Autodesk Inventor part; units mm, degrees
ref_plane "YZ Plane" through (0, 0, 0) normal (1, 0, 0) x (0, 1, 0)
ref_plane "XZ Plane" through (0, 0, 0) normal (0, 1, 0) x (-1, 0, 0)
ref_plane "XY Plane" through (0, 0, 0) normal (0, 0, 1) x (1, 0, 0)
sketch "Sketch1" plane through (0, 0, 0) normal (1, 0, 0) x (0, 1, 0)
  line L0 (6.1324, -19.2794) -> (-5.8676, -19.2794)
  line L1 (-5.8676, -19.2794) -> (-5.8676, -43.2794)
  line L2 (-5.8676, -43.2794) -> (6.1324, -43.2794)
  line L3 (6.1324, -43.2794) -> (6.1324, -19.2794)
  point P0 (0, 0)
  dimension "d0" = 12
  dimension "d1" = 24
extrude "Extrusion1" add sketch "Sketch1" along normal blind 1.8
sketch "Sketch2" plane through (1.8, 0, 0) normal (1, 0, 0) x (0, 0, -1)
  circle A0 centre (38.2794, 0.1324) radius 3.5
  line L0 (43.2794, -5.8676) -> (43.2794, 6.1324)
  line L1 (19.2794, -5.8676) -> (43.2794, -5.8676)
  point P0 (0, 0)
  dimension "d4" = 7
  dimension "d5" = 5
  dimension "d6" = 6
extrude "Extrusion2" cut sketch "Sketch2" against normal blind 0.8
sketch "Sketch3" plane through (1.8, 0, 0) normal (1, 0, 0) x (0, 0, -1)
  line L0 (19.2794, 6.1324) -> (19.2794, -5.8676)
  line L1 (43.2794, -5.8676) -> (43.2794, 6.1324)
  line L2 (19.2794, 6.1324) -> (43.2794, 6.1324)
  line L3 (43.2794, 6.1324) -> (43.2794, -5.8676)
  line L4 (43.2794, -5.8676) -> (19.2794, -5.8676)
  line L5 (19.2794, -5.8676) -> (19.2794, 6.1324)
  circle A0 centre (38.2794, 0.1324) radius 3.5
  circle A1 centre (38.2794, 0.1324) radius 3.5
  point P0 (0, 0)
  point P1 (43.2794, 6.1324)
extrude "Extrusion3" add sketch "Sketch3" along normal blind 2.5
sketch "Sketch4" plane through (4.3, 0, 0) normal (1, 0, 0) x (0, 0, -1)
  circle A0 centre (38.2794, 0.1324) radius 3.5
  line L0 (36.7494, 3.2802) -> (22.2595, 1.8824)
  line L1 (36.7494, -3.0155) -> (22.2595, -1.6176)
  arc A1 (22.2595, 1.8824) -> (22.2595, -1.6176) centre (25.2089, 0.1324) ccw
  line L2 (43.2794, 6.1324) -> (19.2794, 6.1324)
  point P0 (0, 0)
  point P1 (21.7794, 0.1324)
  dimension "d15" = 1.53
  dimension "d16" = 1.53
  dimension "d17" = 16.5
  dimension "d18" = 3.5
  dimension "d19" = 6
extrude "Extrusion4" cut sketch "Sketch4" against normal blind 2.5 contours A0 L1 A1 L0
sketch "Sketch5" plane through (0, 0, 0) normal (-1, 0, 0) x (0, 0, 1)
  circle A0 centre (-38.2794, 0.1324) radius 3.5
  circle A1 centre (-38.2794, 0.1324) radius 1.25
  point P0 (0, 0)
  dimension "d22" = 2.5
extrude "Extrusion5" cut sketch "Sketch5" against normal blind 2.5 contours A1
sketch "Sketch6" plane through (4.3, 0, 0) normal (1, 0, 0) x (0, 0, -1)
  line L0 (43.2794, 6.1324) -> (19.2794, 6.1324)
  line L1 (19.2794, -5.8676) -> (43.2794, -5.8676)
  line L2 (19.2794, 6.1324) -> (22.2794, 6.1324)
  line L3 (22.2794, 6.1324) -> (22.2794, -5.8676)
  line L4 (22.2794, -5.8676) -> (19.2794, -5.8676)
  line L5 (19.2794, -5.8676) -> (19.2794, 6.1324)
  point P0 (0, 0)
  point P1 (22.2794, 6.1324)
  dimension "d25" = 3
extrude "Extrusion6" add sketch "Sketch6" along normal blind 45.5
sketch "Sketch7" plane through (0, -5.8676, -19.2794) normal (0, 0, 1) x (1, 0, 0)
  circle A0 centre (39.861, 6) radius 1.5
  line L0 (49.8, 12) -> (49.8, 0)
  line L1 (0, 12) -> (49.8, 12)
  line L2 (0, 12) -> (0, 0)
  point P0 (0, 5.8676)
  dimension "d28" = 3
  dimension "d30" = 6
  dimension "d38" = 39.861
extrude "Extrusion7" cut sketch "Sketch7" against normal blind 40
sketch "Sketch8" plane through (1.8, 0, 0) normal (1, 0, 0) x (0, 0, -1)
  circle A0 centre (25.7794, 0.1324) radius 1
  circle A1 centre (38.2794, 0.1324) radius 1.25
  point P0 (0, 0)
  dimension "d33" = 2
  dimension "d34" = 12.5
  dimension "d35" = 0
extrude "Extrusion8" cut sketch "Sketch8" against normal blind 10 contours A0
properties part number "18_2"
Part model, mm, in its own coordinate system. A direction names the side the tool comes from. Round coordinates to 2 decimals unless told otherwise and drop trailing zeros. Loops run counter-clockwise (first coordinate to the right, second up) from the corner with the lowest first, then second, coordinate; pieces in that order, holes last. Notation, with made-up numbers: (-20.5, -15.5) -> (22.5, -15.5) arc R25 cw to (22.5, 15.5) -> close; hole circle Ø11 at (19.25, -18). An arc over 180 degrees is marked (long way). Use CSV: the item, a comma, the result in double quotes. Start each with the question number.
1) Wall check: L1, parallel to X at y = -4, z = -38.75; L2, parallel to Z at x = 32.5, y = 0; L3, parallel to X at y = -1.25, z = -28. Give the ranges that are in metal, low to high. Write a range as [from, to].
2) Cut at B-B, the plane x = 40.5. Write the cut outline in (y, z).
3) Pull direction Y, two halves, no side cores. Call faces 5 (the flat face through (25, 0, -19.279)), 6 (the flat face through (17, -5.868, -21)), 7 (the cylindrical face through (0.493, 0.508, -37.087)): +Y half, -Y half, draft (parallel to the pull), parting line (faces both ways), or undercut.
4) Cut at C-C, the plane z = -27.5. Write the cut outline in (x, y).
5) Drop flat-ended pins along their axis: P1, Ø1.8, axis at x = 39.86, y = 0.13, coming from the +Z side; P2, Ø2, axis at y = 2, z = -32.5, coming from the +X side; P3, Ø3, axis at y = 0.13, z = -25.78, coming from the +X side; P4, Ø3, axis at y = 0.13, z = -38.28, coming from the +X side. Give the stop position or say it passes through.
6) Cut at A-A, the plane z = -39. Write the cut outline in (x, y).
7) Which spindle directions (+Z, -Z, +X, -X, +Y, -Y) get a long thin tool onto all of the face, cutting with end or side? Do faces 1 (the flat face through (16, 6.132, -22)), 2 (the cylindrical face through (2.627, -0.919, -41.618)), 3 (the flat face through (27, 0, -22.279)), 4 (the cylindrical face through (3.07, 0.16, -21.78)). Say none if no direction does.
Determined:
1,L1,"x = [0, 4.3]"
1,L2,"z = [-22.28, -19.28]"
1,L3,"x = [0, 1.8]"
2,outline,"(-5.87, -22.28) -> (-1.22, -22.28) -> (-1.22, -19.28) -> (-5.87, -19.28) -> close; (1.49, -22.28) -> (6.13, -22.28) -> (6.13, -19.28) -> (1.49, -19.28) -> close"
3,face 5,"draft"
3,face 6,"-Y half"
3,face 7,"undercut"
4,outline,"(0, -5.87) -> (4.3, -5.87) -> (4.3, -2.12) -> (1.8, -2.12) -> (1.8, 2.39) -> (4.3, 2.39) -> (4.3, 6.13) -> (0, 6.13) -> close"
5,P1,"passes through"
5,P2,"stops at x = 4.3"
5,P3,"stops at x = 1.8"
5,P4,"stops at x = 1"
6,outline,"(0, -5.87) -> (4.3, -5.87) -> (4.3, -3.29) -> (1, -3.29) -> (1, -0.89) -> (0, -0.89) -> close; (0, 1.15) -> (1, 1.15) -> (1, 3.56) -> (4.3, 3.56) -> (4.3, 6.13) -> (0, 6.13) -> close"
7,face 1,"+Z, -Z, +X, -X, +Y"
7,face 2,"+X"
7,face 3,"-Z, +X, +Y, -Y"
7,face 4,"none"
